Geometry: final body of the model. Coordinates: model frame, mm. Face numbers are marked on the shaded views. A direction names the side the tool comes from. Give positions to 0.01 mm unless a question says otherwise; leave off trailing zeros. Write each loop counter-clockwise with the first axis right and the second up, starting at its lowest first coordinate (ties: lowest second). Pieces come first, ordered by that corner, then holes. Notation, with made-up numbers: (55, 78.25) -> (76, 78.25) arc R19 cw to (76, 89.25) -> close; hole circle Ø5 at (57, 55.5). An arc over 180 degrees is marked (long way). Answer as a JSON object with one key per item and string values.
from build123d import *

# Parameters (mm, degrees)
F0_W      = 21
F0_H      = 20
F1_DEPTH  = 3
F2_W      = 2.85
F2_H      = 20
F3_DEPTH  = 12
F4_R      = 6
F5_R      = 1.75
F6_DEPTH  = 21.001
F7_R      = 5
F8_R      = 1.75
F9_DEPTH  = 3.001
F10_DEPTH = 2
F12_DEPTH = 2.5
F13_R     = 2.875
F14_DEPTH = 1


with BuildPart() as f1:
    # F0 (on Top) → F1 (new body)
    with BuildSketch(Plane.XY):
        with Locations((10.5, 10)):
            Rectangle(F0_W, F0_H)
    extrude(amount=F1_DEPTH)

    # F2 (on face) → F3 (join)
    with BuildSketch(Plane.XY.offset(3)):
        with Locations((1.425, 10)):
            Rectangle(F2_W, F2_H)
        with Locations((19.575, 10)):
            Rectangle(F2_W, F2_H)
    extrude(amount=F3_DEPTH)

    # F4
    f4_edges = [f1.edges().sort_by_distance(p)[0] for p in [
        (0, 0, 7.5),
    ]]
    fillet(f4_edges, radius=F4_R)

    # F5 (on face) → F6 (cut, through all)
    with BuildSketch(Plane(origin=(0, 0, 0), x_dir=(0, -1, 0), z_dir=(-1, 0, 0))):
        with Locations((-15, 10)):
            Circle(F5_R)
        Polygon((0, 15), (-10, 15), (0, 3), align=None)
    extrude(amount=-F6_DEPTH, mode=Mode.SUBTRACT)

    # F7
    f7_edges = [f1.edges().sort_by_distance(p)[0] for p in [
        (1.425, 20, 15),
        (19.575, 20, 15),
        (1.425, 10, 15),
        (19.575, 10, 15),
    ]]
    fillet(f7_edges, radius=F7_R)

    # F8 (on face) → F9 (cut, through all)
    with BuildSketch(Plane.XY.offset(3)):
        with Locations((6, 6)):
            Circle(F8_R)
        with Locations((15, 6)):
            Circle(F8_R)
    extrude(amount=-F9_DEPTH, mode=Mode.SUBTRACT)

    # F10 (add): a face of the model
    f10_faces = [f1.faces().sort_by_distance(p)[0] for p in [
        (21, 11.3560605972, 6.2794868265),
    ]]
    extrude(f10_faces, amount=F10_DEPTH)

    # F11 (on face) → F12 (cut)
    with BuildSketch(Plane.YZ.offset(23)):
        Polygon((17.85, 8.3545517328), (17.85, 11.6454482672), (15, 13.2908965344), (12.15, 11.6454482672), (12.15, 8.3545517328), (15, 6.7091034656), align=None)
    extrude(amount=-F12_DEPTH, mode=Mode.SUBTRACT)

    # F13 (on face) → F14 (cut)
    with BuildSketch(Plane.XY.offset(3)):
        with Locations((6, 6)):
            Circle(F13_R)
        with Locations((15, 6)):
            Circle(F13_R)
    extrude(amount=-F14_DEPTH, mode=Mode.SUBTRACT)


solid = f1.part
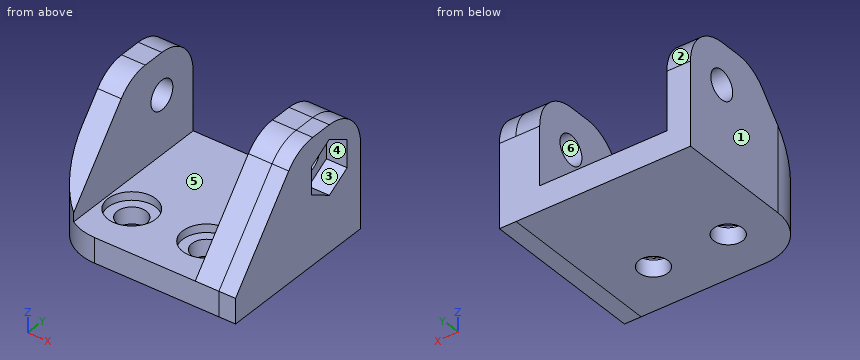
Q1. Cut plane B-B (z = 7). Return the cut outline in (x, y), and give its area (3 significant figures).
Values:
{"outline": "(0, 6) arc R6 ccw to (0.63, 3.33) -> (2.85, 3.33) -> (2.85, 20) -> (0, 20) -> close; (18.15, 3.33) -> (23, 3.33) -> (23, 14.5) -> (20.5, 14.5) -> (20.5, 15.5) -> (23, 15.5) -> (23, 20) -> (18.15, 20) -> close", "area": "125 mm²"}
Q2. First-contact query: P1, Ø1, axis at x = 4, y = 4.5, coming from the +Z side; P2, Ø3, axis at x = 21.5, z = 9.5, coming from the -Y side; P3, Ø4.5, axis at y = 15, z = 10, coming from the +X side. Flat tips, straight axial feed; report the tip coordinate or a pass-through.
Values:
{"P1": "z = 3", "P2": "y = 4.17", "P3": "x = 20.5"}
Q3. Cut plane D-D (z = 9). Return the cut outline in (x, y).
Values:
{"outline": "(0, 6) arc R6 ccw to (0.08, 5) -> (2.85, 5) -> (2.85, 13.56) -> (0, 13.56) -> close; (0, 16.44) -> (2.85, 16.44) -> (2.85, 20) -> (0, 20) -> close; (18.15, 5) -> (23, 5) -> (23, 12.15) -> (20.5, 12.15) -> (20.5, 13.56) -> (18.15, 13.56) -> close; (18.15, 16.44) -> (20.5, 16.44) -> (20.5, 17.85) -> (23, 17.85) -> (23, 20) -> (18.15, 20) -> close"}
Q4. Material intervals for L1, parallel to X at y = 7, z = 4.25; L2, parallel to Y at x = 6, z = 1; L3, parallel to Y at x = 15, z = 2.4 (3 decimals), sorted ascending. Write a range as from..to.
Values:
{"L1": "0..2.85, 18.15..23", "L2": "0..4.25, 7.75..20", "L3": "0..3.125, 8.875..20"}
Q5. Mould query, pull axis Z, two halves, no side actions, for the marked faces 1, 2 and 3. Classes: pulls with the +Z half, pulls with the -Z half, needs draft (parallel to the pull), parting line crosses it, or undercut.
Values:
{"face 1": "needs draft", "face 2": "pulls with the +Z half", "face 3": "undercut"}
Q6. Set-up query: the marked faces 4, 5 and 6. Return all of +Z, -Z, +X, -X, +Y, -Y with unobstructed straight access to the full face (end or side cutting, diameter ignored); none if empty.
Values:
{"face 4": "+X", "face 5": "+Z, +Y, -Y", "face 6": "+X, -X"}
Q7. Cut plane A-A (z = 2.5). Return the cut outline in (x, y) (3 decimals).
Values:
{"outline": "(0, 6) arc R6 ccw to (6, 0) -> (23, 0) -> (23, 20) -> (0, 20) -> close; hole circle Ø5.75 at (6, 6); hole circle Ø5.75 at (15, 6)"}
Q8. Cut plane C-C (x = 2.5). Return the cut outline in (y, z), and give its area (3 significant figures).
Values:
{"outline": "(1.13, 0) -> (20, 0) -> (20, 10) arc R5 ccw to (15, 15) -> (12.34, 15) arc R5 ccw to (8.5, 13.2) -> (1.13, 4.35) -> close; hole circle Ø3.5 at (15, 10)", "area": "220 mm²"}
